Model file for the job. Use its own axes, mm. Face numbers are marked on the shaded views. Coordinates: 2 decimals unless noted, no trailing zeros. Order: outer loops, then holes, each group sorted by start corner. A loop starts at its lowest first (then second) coordinate and runs counter-clockwise, first axis right, second up. Notation, with made-up numbers: (-24, 89.25) -> (-1, 89.25) arc R22 cw to (-1, 122.25) -> close; hole circle Ø11 at (28, -20.5). An arc over 180 degrees is marked (long way). Return JSON: item names as keys, results as strings. Group by question number.
1) Cut at C-C (z = 59.5). Write the cut outline in (x, y).
2) Cut at D-D (y = -90). Write the cut outline in (x, z), and give its area (3 significant figures).
3) Flat gauge pins, fed straight in: pin 1 (1.3 mm diameter, centred on y = 18, z = 7, fed in from -X); pin 2 (4 mm diameter, centred on x = 55.5, y = 29.5, fed in from +Z); pin 3 (2.5 mm diameter, centred on x = 0, z = 13, fed in from -Y). Where does each tip first touch, or does it go through?
4) Cut at A-A (y = 0). Write the cut outline in (x, z), and give its area (3 significant figures).
5) Cut at B-B (x = 11). Write the cut outline in (y, z).
6) Probe line 1 (Y direction, x = 0, z = 13.75); line 2 (Z direction, x = 28, y = -45.5). List the from-to ranges inside material, lowest first.
7) Pull direction X, two halves, no side cores. Call the marked faces 1, 2 and 3: +X half, -X half, draft (parallel to the pull), parting line (faces both ways), or undercut.
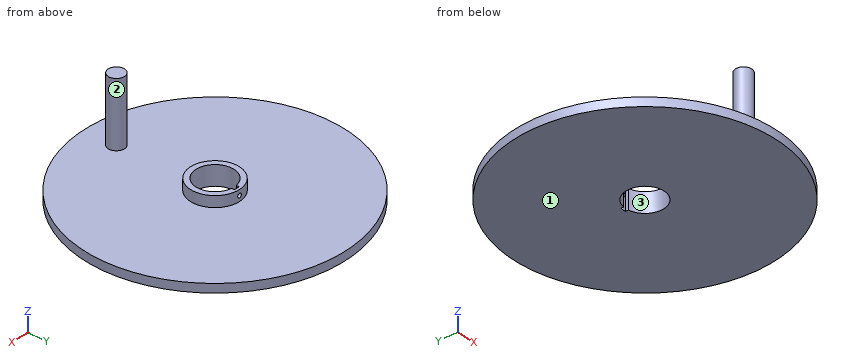
from build123d import *

# Parameters (mm, degrees)
SKETCH1_R           = 120
BOSS_EXTRUDE1_DEPTH = 8
SKETCH2_R           = 22.5
BOSS_EXTRUDE2_DEPTH = 10
SKETCH3_R           = 2
CUT_EXTRUDE1_DEPTH  = 25
SKETCH4_R           = 7.5
BOSS_EXTRUDE3_DEPTH = 60


with BuildPart() as part:
    # Sketch1 → Boss-Extrude1 (new body)
    with BuildSketch(Plane.XY):
        Circle(SKETCH1_R)
        with BuildLine():
            Line((-2.5, 20), (2.5, 20))
            Line((2.5, 20), (2.5, 17.320508076))
            ThreePointArc((2.5, 17.320508076), (0, -17.5), (-2.5, 17.320508076))
            Line((-2.5, 17.320508076), (-2.5, 20))
        make_face(mode=Mode.SUBTRACT)
    extrude(amount=BOSS_EXTRUDE1_DEPTH)

    # Sketch2 → Boss-Extrude2 (add)
    with BuildSketch(Plane.XY.offset(8)):
        Circle(SKETCH2_R)
        with BuildLine():
            Line((-2.5, 17.320508076), (-2.5, 20))
            Line((-2.5, 20), (2.5, 20))
            Line((2.5, 20), (2.5, 17.320508076))
            ThreePointArc((2.5, 17.320508076), (0, -17.5), (-2.5, 17.320508076))
        make_face(mode=Mode.SUBTRACT)
    extrude(amount=BOSS_EXTRUDE2_DEPTH)

    # Sketch3 → Cut-Extrude1 (cut)
    with BuildSketch(Plane(origin=(0, 0, 0), x_dir=(1, 0, 0), z_dir=(0, 1, 0))):
        with Locations(Location((0, -13, 0), (0, 0, 90))):
            Circle(SKETCH3_R)
    extrude(amount=CUT_EXTRUDE1_DEPTH, mode=Mode.SUBTRACT)

    # Sketch4 → Boss-Extrude3 (add)
    with BuildSketch(Plane.XY.offset(8)):
        with Locations((0, -90)):
            Circle(SKETCH4_R)
    extrude(amount=BOSS_EXTRUDE3_DEPTH)


solid = part.part
Answers below:
{
 "1": {"outline": "circle Ø15 at (0, -90)"},
 "2": {"outline": "(-79.37, 0) -> (79.37, 0) -> (79.37, 8) -> (7.5, 8) -> (7.5, 68) -> (-7.5, 68) -> (-7.5, 8) -> (-79.37, 8) -> close", "area": "2,170 mm^2"},
 "3": {"pin 1": "stops at x = -118.74", "pin 2": "stops at z = 8", "pin 3": "stops at y = -97.5"},
 "4": {"outline": "(-120, 0) -> (-17.5, 0) -> (-17.5, 18) -> (-22.5, 18) -> (-22.5, 8) -> (-120, 8) -> close; (17.5, 0) -> (120, 0) -> (120, 8) -> (22.5, 8) -> (22.5, 18) -> (17.5, 18) -> close", "area": "1,740 mm^2"},
 "5": {"outline": "(-119.49, 0) -> (-13.61, 0) -> (-13.61, 18) -> (-19.63, 18) -> (-19.63, 8) -> (-119.49, 8) -> close; (13.61, 0) -> (119.49, 0) -> (119.49, 8) -> (19.63, 8) -> (19.63, 18) -> (13.61, 18) -> close"},
 "6": {"line 1": "y = -97.5 to -82.5, -22.5 to -17.5", "line 2": "z = 0 to 8"},
 "7": {"face 1": "draft", "face 2": "parting line", "face 3": "undercut"}
}
